Part print with two shaded views. Sizes in mm from the minimum x, y, z corner. A direction names the side the tool comes from. Round coordinates to 2 decimals unless told otherwise and drop trailing zeros. Loops run counter-clockwise (first coordinate to the right, second up) from the corner with the lowest first, then second, coordinate; pieces in that order, holes last. Notation, with made-up numbers: (60.5, -21.5) -> (104.5, -21.5) arc R24 ccw to (104.5, -11.5) -> close; hole circle Ø10 at (79.5, 52). An arc over 180 degrees is marked (long way). Use a Markdown table: item, result. Add a question column.
Item 1: Flat gauge pins, fed straight in: pin 1 (4 mm diameter, centred on x = 39.55, z = 3.63, fed in from +Y); pin 2 (10 mm diameter, centred on x = 36.5, y = 56.5, fed in from +Z). Where does each tip first touch, or does it go through?
Item 2: Cut at C-C, the plane x = 21.59. List the corners of the cut face in (y, z), plus the area to 3 significant figures.
Item 3: Cut at B-B, the plane x = 4. List the corners of the cut face in (y, z) (1 decimal).
Item 4: Cut at A-A, the plane z = 21.59. List the corners of the cut face in (x, y).
Item 5: Cut at D-D, the plane y = 61. List the corners of the cut face in (x, z).
Item 6: Probe line 1 (Z direction, x = 39.5, y = 21.5) (1 decimal); line 2 (Y direction, x = 33.5, z = 33.5); line 3 (Z direction, x = 39, y = 20.5) (1 decimal). List the from-to ranges inside material, lowest first. Write a range as [from, to].
Item 7: Which spindle directions (+Z, -Z, +X, -X, +Y, -Y) get a long thin tool onto all of the face, cutting with end or side? Do the marked faces 1 and 2. Say none if no direction does.
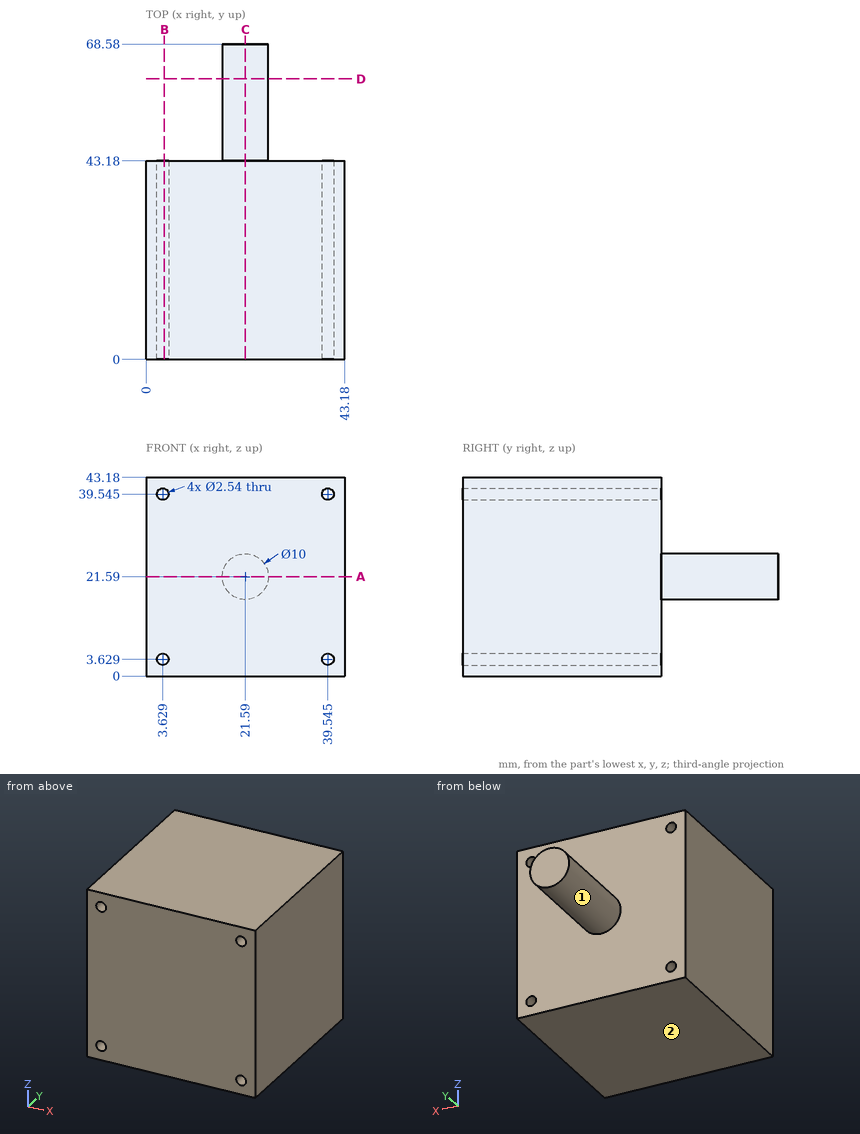
A:
| question | item | result |
|---|---|---|
| 1 | pin 1 | stops at y = 43.18 |
| 1 | pin 2 | passes through |
| 2 | outline | (0, 0) -> (43.18, 0) -> (43.18, 16.59) -> (68.58, 16.59) -> (68.58, 26.59) -> (43.18, 26.59) -> (43.18, 43.18) -> (0, 43.18) -> close |
| 2 | area | 2,120 mm^2 |
| 3 | outline | (0, 0) -> (43.2, 0) -> (43.2, 2.4) -> (0, 2.4) -> close; (0, 4.8) -> (43.2, 4.8) -> (43.2, 38.3) -> (0, 38.3) -> close; (0, 40.8) -> (43.2, 40.8) -> (43.2, 43.2) -> (0, 43.2) -> close |
| 4 | outline | (0, 0) -> (43.18, 0) -> (43.18, 43.18) -> (26.59, 43.18) -> (26.59, 68.58) -> (16.59, 68.58) -> (16.59, 43.18) -> (0, 43.18) -> close |
| 5 | outline | circle Ø10 at (21.59, 21.59) |
| 6 | line 1 | z = [0, 2.4], [4.9, 38.3], [40.8, 43.2] |
| 6 | line 2 | y = [0, 43.18] |
| 6 | line 3 | z = [0, 2.5], [4.8, 38.4], [40.7, 43.2] |
| 7 | face 1 | +Y |
| 7 | face 2 | -Z, +X, -X, +Y, -Y |
